Model file for the job. Use its own axes, mm. Face numbers are marked on the shaded views. A direction names the side the tool comes from. Round coordinates to 2 decimals unless told otherwise and drop trailing zeros. Loops run counter-clockwise (first coordinate to the right, second up) from the corner with the lowest first, then second, coordinate; pieces in that order, holes last. Notation, with made-up numbers: M 10.5,-21 L 43.5,-21 A16 cw 43.5,-5 Z; hole C 0,-23 d10. An arc over 180 degrees is marked long. Use a Markdown table: item, result. Add a question column.
Q1. Probe line 1 (X direction, y = 11, z = -17.5); line 2 (X direction, y = 12, z = -2); line 3 (Z direction, x = -13, y = 8). List the from-to ranges inside material, lowest first. Write a range as from..to.
Q2. Pin check, flat tips, straight feed: pin 1 (4 mm diameter, centred on x = -17.5, y = 4.5, fed in from +Z); pin 2 (3 mm diameter, centred on x = -3, z = -31, fed in from +Y); pin 3 (7.5 mm diameter, centred on x = 2.5, y = 10, fed in from +Z). Stop position of each tip, or through.
Q3. Mould opens along X. For the marked faces 1, 2, 3 and 4 say: +X half, -X half, draft (parallel to the pull), parting line (faces both ways), or undercut.
Q4. Cut at C-C (z = -14). Give the cut face in (x, y).
Q5. Cut at A-A (z = -22.5). Give the cut face in (x, y), plus the area to 3 significant figures.
Q6. Cut at D-D (x = 5.5). Give the cut face in (y, z), plus the area to 3 significant figures.
Q7. Cut at B-B (y = 1.5). Give the cut face in (x, z), plus the area to 3 significant figures.
Q8. Tool access for the marked faces 5 and 6: list every direction of +Z, -Z, +X, -X, +Y, -Y with a clear straight run to the whole face (end or side of a thin tool).
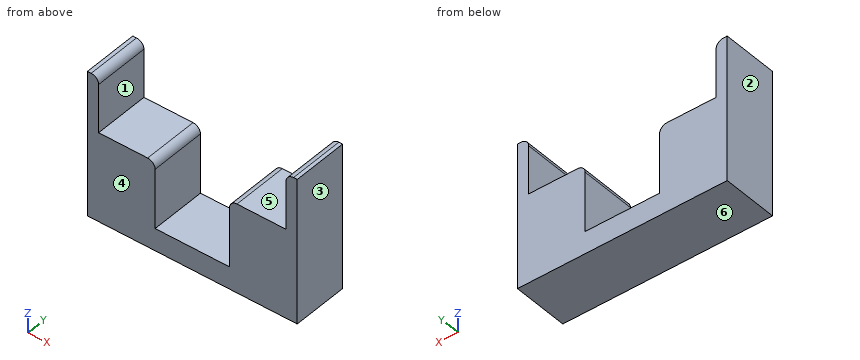
from build123d import *

# Parameters (mm, degrees)
BOSS_EXTRUDE1_DEPTH = 15
FILLET2_R           = 2


with BuildPart() as part:
    # Sketch1 → Boss-Extrude1 (new body)
    with BuildSketch(Plane(origin=(0, 0, 0), x_dir=(1, 0, 0), z_dir=(0, 1, 0))):
        Polygon((26.949275536, 0.12972973), (29.949275536, 0.12972973), (29.949275536, 39.12972973), (-26.450724464, 39.12972973), (-26.450724464, 0.12972973), (-23.450724464, 0.12972973), (-23.450724464, 15.12972973), (-8.250724464, 15.12972973), (-8.250724464, 33.12972973), (11.749275536, 33.12972973), (11.749275536, 15.12972973), (26.949275536, 15.12972973), align=None)
    extrude(amount=BOSS_EXTRUDE1_DEPTH)

    # Fillet2
    fillet2_edges = [part.edges().sort_by_distance(p)[0] for p in [
        (26.949275536, 7.5, -0.12972973),
        (11.749275536, 7.5, -15.12972973),
        (-8.250724464, 7.5, -15.12972973),
        (-23.450724464, 7.5, -0.12972973),
    ]]
    fillet(fillet2_edges, radius=FILLET2_R)


solid = part.part
Checked values:
| question | item | result |
|---|---|---|
| 1 | line 1 | x = -26.45..-8.25, 11.75..29.95 |
| 1 | line 2 | x = -26.45..-23.45, 26.95..29.95 |
| 1 | line 3 | z = -39.13..-15.13 |
| 2 | pin 1 | stops at z = -15.13 |
| 2 | pin 2 | passes through |
| 2 | pin 3 | stops at z = -33.13 |
| 3 | face 1 | undercut |
| 3 | face 2 | -X half |
| 3 | face 3 | +X half |
| 3 | face 4 | draft |
| 4 | outline | M -26.45,0 L -23.45,0 L -23.45,15 L -26.45,15 Z; M 26.95,0 L 29.95,0 L 29.95,15 L 26.95,15 Z |
| 5 | outline | M -26.45,0 L -8.25,0 L -8.25,15 L -26.45,15 Z; M 11.75,0 L 29.95,0 L 29.95,15 L 11.75,15 Z |
| 5 | area | 546 mm^2 |
| 6 | outline | M 0,-39.13 L 15,-39.13 L 15,-33.13 L 0,-33.13 Z |
| 6 | area | 90.0 mm^2 |
| 7 | outline | M -26.45,-39.13 L 29.95,-39.13 L 29.95,-0.13 L 28.95,-0.13 A2 ccw 26.95,-2.13 L 26.95,-15.13 L 13.75,-15.13 A2 ccw 11.75,-17.13 L 11.75,-33.13 L -8.25,-33.13 L -8.25,-17.13 A2 ccw -10.25,-15.13 L -23.45,-15.13 L -23.45,-2.13 A2 ccw -25.45,-0.13 L -26.45,-0.13 Z |
| 7 | area | 1,080 mm^2 |
| 8 | face 5 | +Z, +Y, -Y |
| 8 | face 6 | -Z, +X, -X, +Y, -Y |
